For this review, take the finished solid that the model builds, in its own axes (mm). Coordinates: 2 decimals unless noted, no trailing zeros. Write each loop counter-clockwise with the first axis right and the second up, starting at its lowest first coordinate (ties: lowest second). Pieces come first, ordered by that corner, then holes.
1) We need section D-D on x = -0.25. Write out the cut boundary in (y, z).
2) To check wall thickness, follow line 1 along X through (y, z) = (9.5, 0.4); line 2 along X through (y, z) = (-9.5, 0.3). State the ranges of each line that lie inside material, in increasing order.
3) We need section C-C on y = 8.5. Write out the cut boundary in (x, z).
4) We need section A-A on x = 2.5. Write out the cut boundary in (y, z).
5) Mouldability with a two-part tool opening along Y and no side actions: class faces 1 (the face through (-11.5, 0.1, 0.5)), 2 (the face through (10.7, 10.4, 0.5)), 3 (the face through (-2.381, -8.963, 0.507)), 4 (the face through (-10.9, 10.93, 0.49)) as pulls with the +Y half, pulls with the -Y half, needs draft (parallel to the pull), parting line crosses it, or undercut.
6) We need section B-B on z = 0.55. Write out the cut boundary in (x, y).
from build123d import *

# Parameters (mm, degrees)
F1_DEPTH = 1
F2_D     = 3
F3_D     = 1.1


with BuildPart() as f1:
    # F0 (on Top) → F1 (new body)
    with BuildSketch(Plane.XY):
        with BuildLine():
            Line((-9.5, -11.5), (9.5, -11.5))
            ThreePointArc((9.5, -11.5), (10.9142135624, -10.9142135624), (11.5, -9.5))
            Line((11.5, -9.5), (11.5, 9.5))
            ThreePointArc((11.5, 9.5), (10.9142135624, 10.9142135624), (9.5, 11.5))
            Line((9.5, 11.5), (-9.5, 11.5))
            ThreePointArc((-9.5, 11.5), (-10.9142135624, 10.9142135624), (-11.5, 9.5))
            Line((-11.5, 9.5), (-11.5, -9.5))
            ThreePointArc((-11.5, -9.5), (-10.9142135624, -10.9142135624), (-9.5, -11.5))
        make_face()
    extrude(amount=F1_DEPTH)

    # F2 (through all)
    with Locations(Plane(origin=(0, 0, 0), x_dir=(1, 0, 0), z_dir=(0, 0, -1))):
        with Locations((-9.5, -9.5), (9.5, -9.5), (9.5, 9.5), (-9.5, 9.5)):
            Hole(F2_D / 2)

    # F3 (through all)
    with Locations(Plane(origin=(0, 0, 0), x_dir=(1, 0, 0), z_dir=(0, 0, -1))):
        with Locations((-2.5, 9.5), (0, 9.5), (2.5, 9.5)):
            Hole(F3_D / 2)


solid = f1.part
Result:
1. outline: (-11.5, 0) - (-9.99, 0) - (-9.99, 1) - (-11.5, 1) - close; (-9.01, 0) - (11.5, 0) - (11.5, 1) - (-9.01, 1) - close
2. line 1: x = -11.5 to -11, -8 to 8, 11 to 11.5
2. line 2: x = -11.5 to -11, -8 to -3.05, -1.95 to -0.55, 0.55 to 1.95, 3.05 to 8, 11 to 11.5
3. outline: (-11.5, 0) - (-10.62, 0) - (-10.62, 1) - (-11.5, 1) - close; (-8.38, 0) - (8.38, 0) - (8.38, 1) - (-8.38, 1) - close; (10.62, 0) - (11.5, 0) - (11.5, 1) - (10.62, 1) - close
4. outline: (-11.5, 0) - (-10.05, 0) - (-10.05, 1) - (-11.5, 1) - close; (-8.95, 0) - (11.5, 0) - (11.5, 1) - (-8.95, 1) - close
5. face 1: needs draft
5. face 2: undercut
5. face 3: undercut
5. face 4: pulls with the +Y half
6. outline: (-11.5, -9.5) arc R2 ccw to (-9.5, -11.5) - (9.5, -11.5) arc R2 ccw to (11.5, -9.5) - (11.5, 9.5) arc R2 ccw to (9.5, 11.5) - (-9.5, 11.5) arc R2 ccw to (-11.5, 9.5) - close; hole circle Ø3 at (-9.5, -9.5); hole circle Ø3 at (-9.5, 9.5); hole circle Ø1.1 at (-2.5, -9.5); hole circle Ø1.1 at (0, -9.5); hole circle Ø1.1 at (2.5, -9.5); hole circle Ø3 at (9.5, -9.5); hole circle Ø3 at (9.5, 9.5)
